Could you check a few things on this model? Use its own coordinates, in mm. A direction names the side the tool comes from. Give positions to 0.01 mm unless a question says otherwise; leave off trailing zeros. Loops run counter-clockwise (first coordinate to the right, second up) from the corner with the lowest first, then second, coordinate; pieces in that order, holes last. Notation, with made-up numbers: (13, 15) - (58, 15) arc R16 ccw to (58, 39) - close; hole circle Ø9 at (6.25, 37). An arc over 180 degrees is marked (long way). Use CSV: the item, a comma, the result in double quotes.
from build123d import *

# Parameters (mm, degrees)
SKETCH_1_W          = 45
SKETCH_1_H          = 39
EXTRUDE_1_DEPTH     = 15
CUT_EXTRUDE_1_DEPTH = 11
SKETCH_3_R          = 1.85
CUT_EXTRUDE_2_DEPTH = 3
SKETCH_4_R          = 1.25
CUT_EXTRUDE_3_DEPTH = 40.575876491
SKETCH_5_R          = 8
CUT_EXTRUDE_4_DEPTH = 12
SKETCH_6_R          = 2.5
EXTRUDE_2_DEPTH     = 1
SKETCH_7_R          = 1.5
EXTRUDE_3_DEPTH     = 1.8
SKETCH_8_W          = 45
SKETCH_8_H          = 15
EXTRUDE_4_DEPTH     = 6
SKETCH_10_R         = 1.5
CUT_EXTRUDE_5_DEPTH = 38.16853512
CUT_EXTRUDE_6_DEPTH = 8.3
SKETCH_12_R         = 4.25
CUT_EXTRUDE_7_DEPTH = 38.16853508
CHAMFER_4_SIZE      = 2
CHAMFER_2_SIZE      = 0.5
CHAMFER_3_SIZE      = 1


with BuildPart() as part:
    # 草图1 → 凸台-拉伸1 (new body)
    with BuildSketch(Plane(origin=(0, 0, 0), x_dir=(1, 0, 0), z_dir=(0, 1, 0))):
        Rectangle(SKETCH_1_W, SKETCH_1_H)
    extrude(amount=EXTRUDE_1_DEPTH)

    # 草图2 → 切除-拉伸1 (cut)
    with BuildSketch(Plane.ZY.offset(22.5)):
        Polygon((-8, 13), (-8, 15), (-6, 15), (-6, 13), (-2.5, 13), (-2.5, 5.65), (-11.5, 5.65), (-11.5, 13), align=None)
        Polygon((6, 2), (6, 0), (8, 0), (8, 2), (11.5, 2), (11.5, 9.35), (2.5, 9.35), (2.5, 2), align=None)
    cut_extrude_1 = extrude(amount=-CUT_EXTRUDE_1_DEPTH, mode=Mode.SUBTRACT)

    # 草图3 → 切除-拉伸2 (cut)
    with BuildSketch(Plane.ZY.offset(11.5)):
        with Locations((-7, 9.325)):
            Circle(SKETCH_3_R)
        with Locations((7, 5.675)):
            Circle(SKETCH_3_R)
    cut_extrude_2 = extrude(amount=-CUT_EXTRUDE_2_DEPTH, mode=Mode.SUBTRACT)

    # 草图4 → 切除-拉伸3 (cut, through all)
    with BuildSketch(Plane.ZY.offset(8.5)):
        with Locations((-7, 9.325)):
            Circle(SKETCH_4_R)
        with Locations((7, 5.675)):
            Circle(SKETCH_4_R)
    extrude(amount=-CUT_EXTRUDE_3_DEPTH, mode=Mode.SUBTRACT)

    # 镜向1: 切除-拉伸1, 切除-拉伸2 across plane
    add(cut_extrude_1.mirror(Plane(origin=(0, 0, 0), x_dir=(0, 0, 1), z_dir=(1, 0, 0))), mode=Mode.SUBTRACT)
    add(cut_extrude_2.mirror(Plane(origin=(0, 0, 0), x_dir=(0, 0, 1), z_dir=(1, 0, 0))), mode=Mode.SUBTRACT)

    # 草图5 → 切除-拉伸4 (cut)
    with BuildSketch(Plane.XZ):
        with Locations(Location((0, 0, 0), (0, 0, 270))):
            Circle(SKETCH_5_R)
    extrude(amount=-CUT_EXTRUDE_4_DEPTH, mode=Mode.SUBTRACT)

    # 草图6 → 凸台-拉伸2 (add)
    with BuildSketch(Plane.XZ.offset(-12)):
        with Locations(Location((0, 0, 0), (0, 0, 270))):
            Circle(SKETCH_6_R)
    extrude(amount=EXTRUDE_2_DEPTH)

    # 草图7 → 凸台-拉伸3 (add)
    with BuildSketch(Plane.XZ.offset(-11)):
        with Locations(Location((0, 0, 0), (0, 0, 270))):
            Circle(SKETCH_7_R)
    extrude(amount=EXTRUDE_3_DEPTH)

    # 草图8 → 凸台-拉伸4 (add)
    with BuildSketch(Plane.XY.offset(19.5)):
        with Locations((0, 7.5)):
            Rectangle(SKETCH_8_W, SKETCH_8_H)
    extrude(amount=EXTRUDE_4_DEPTH)

    # 草图10 → 切除-拉伸5 (cut, through all)
    with BuildSketch(Plane(origin=(0, 15, 0), x_dir=(1, 0, 0), z_dir=(0, 1, 0))):
        with Locations(Location((-19.5, 16.5, 0), (0, 0, 270))):
            Circle(SKETCH_10_R)
        with Locations(Location((19.5, 16.5, 0), (0, 0, 90))):
            Circle(SKETCH_10_R)
        with Locations(Location((19.5, -22.5, 0), (0, 0, 270))):
            Circle(SKETCH_10_R)
        with Locations(Location((-19.5, -22.5, 0), (0, 0, 90))):
            Circle(SKETCH_10_R)
    extrude(amount=-CUT_EXTRUDE_5_DEPTH, mode=Mode.SUBTRACT)

    # 草图11 → 切除-拉伸6 (cut)
    with BuildSketch(Plane(origin=(0, 15, 0), x_dir=(1, 0, 0), z_dir=(0, 1, 0))):
        with BuildLine():
            Line((-16.5, 16.5), (-16.5, 19.5))
            Line((-16.5, 19.5), (-22.5, 19.5))
            Line((-22.5, 19.5), (-22.5, 13.5))
            Line((-22.5, 13.5), (-19.5, 13.5))
            ThreePointArc((-19.5, 13.5), (-17.378679656, 14.378679656), (-16.5, 16.5))
        make_face()
        with BuildLine():
            Line((22.5, 19.5), (22.5, 13.5))
            Line((22.5, 13.5), (19.5, 13.5))
            ThreePointArc((19.5, 13.5), (17.378679656, 14.378679656), (16.5, 16.5))
            Line((16.5, 16.5), (16.5, 19.5))
            Line((16.5, 19.5), (22.5, 19.5))
        make_face()
        with BuildLine():
            Line((16.5, -25.5), (22.5, -25.5))
            Line((22.5, -25.5), (22.5, -19.5))
            Line((22.5, -19.5), (19.5, -19.5))
            ThreePointArc((19.5, -19.5), (17.378679656, -20.378679656), (16.5, -22.5))
            Line((16.5, -22.5), (16.5, -25.5))
        make_face()
        with BuildLine():
            Line((-22.5, -25.5), (-22.5, -19.5))
            Line((-22.5, -19.5), (-19.5, -19.5))
            ThreePointArc((-19.5, -19.5), (-17.378679656, -20.378679656), (-16.5, -22.5))
            Line((-16.5, -22.5), (-16.5, -25.5))
            Line((-16.5, -25.5), (-22.5, -25.5))
        make_face()
    extrude(amount=-CUT_EXTRUDE_6_DEPTH, mode=Mode.SUBTRACT)

    # 草图12 → 切除-拉伸7 (cut, through all)
    with BuildSketch(Plane.XZ):
        with Locations(Location((0, 17.5, 0), (0, 0, 270))):
            Circle(SKETCH_12_R)
    extrude(amount=-CUT_EXTRUDE_7_DEPTH, mode=Mode.SUBTRACT)

    # 倒角4
    chamfer_4_edges = [part.edges().sort_by_distance(p)[0] for p in [
        (0, 0, 21.75),
    ]]
    chamfer(chamfer_4_edges, length=CHAMFER_4_SIZE)

    # 倒角2
    chamfer_2_edges = [part.edges().sort_by_distance(p)[0] for p in [
        (0, 9.2, 1.5),
    ]]
    chamfer(chamfer_2_edges, length=CHAMFER_2_SIZE)

    # 倒角3
    chamfer_3_edges = [part.edges().sort_by_distance(p)[0] for p in [
        (22.5, 3.35, 25.5),
        (-22.5, 3.35, 25.5),
        (-22.5, 3.35, -19.5),
        (22.5, 3.35, -19.5),
    ]]
    chamfer(chamfer_3_edges, length=CHAMFER_3_SIZE)


solid = part.part
1) Suppose I cut it at D-D (z = -9.5). Please give me the cut outline in (x, y), plus the area to 3 significant figures.
Answer below:
outline,"(-22.5, 0) - (22.5, 0) - (22.5, 5.65) - (11.5, 5.65) - (11.5, 13) - (22.5, 13) - (22.5, 15) - (-22.5, 15) - (-22.5, 13) - (-11.5, 13) - (-11.5, 5.65) - (-22.5, 5.65) - close"
area,"513 mm2"
2) We'd pull the mould along Z, two halves only. Please class faces 1 (the flat face through (0, 8, 25.5)), 2 (the cylindrical face through (4.214, 8.409, 18.053)), 3 (the cylindrical face through (-17.4, 10.91, -14.36)), 4 (the flat face through (22.5, 11, 3)): +Z half, -Z half, draft (parallel to the pull), parting line (faces both ways), or undercut.
Answer below:
face 1,"+Z half"
face 2,"undercut"
face 3,"-Z half"
face 4,"draft"
3) I'm going to push flat-ended pins straight in: P1, Ø1.5, axis at x = 21, y = 12.5, coming from the -Z side; P2, Ø4.5, axis at y = 5.675, z = 7, coming from the -X side; P3, Ø2, axis at y = 9.325, z = -7, coming from the +X side; P4, Ø1, axis at x = 2, z = -3.5, coming from the -Y side. Where does each tip first touch, or does it pass through?
Answer below:
P1,"stops at z = -13.5"
P2,"stops at x = -11.5"
P3,"passes through"
P4,"stops at y = 12"
4) Suppose I cut it at B-B (y = 3). Please give me the cut outline in (x, z).
Answer below:
outline,"(-22.5, -18.5) - (-21.5, -19.5) - (21.5, -19.5) - (22.5, -18.5) - (22.5, 2.5) - (11.5, 2.5) - (11.5, 11.5) - (22.5, 11.5) - (22.5, 24.5) - (21.5, 25.5) - (-21.5, 25.5) - (-22.5, 24.5) - (-22.5, 11.5) - (-11.5, 11.5) - (-11.5, 2.5) - (-22.5, 2.5) - close; hole circle Ø3 at (-19.5, -16.5); hole circle Ø3 at (-19.5, 22.5); hole circle Ø16 at (0, 0); hole circle Ø8.5 at (0, 17.5); hole circle Ø3 at (19.5, -16.5); hole circle Ø3 at (19.5, 22.5)"
5) I need wall thicknesses on line 1 along Z through (x, y) = (14, 7.25); line 2 along X through (y, z) = (1.5, -16.5); line 3 along Z through (x, y) = (-1, 2.25). Which ranges of each line are inside material? Lowest first, please.
Answer below:
line 1,"z = -19.5 to -11.5, -2.5 to 2.5, 11.5 to 25.5"
line 2,"x = -22.5 to -21, -18 to 18, 21 to 22.5"
line 3,"z = -19.5 to -7.94, 7.94 to 13.37, 21.63 to 25.5"
6) Suppose I cut it at C-C (z = 7). Please give me the cut outline in (x, y) (3 decimals).
Answer below:
outline,"(-22.5, 9.35) - (-11.5, 9.35) - (-11.5, 7.525) - (-8.5, 7.525) - (-8.5, 6.925) - (-3.873, 6.925) - (-3.873, 12) - (3.873, 12) - (3.873, 6.925) - (8.5, 6.925) - (8.5, 7.525) - (11.5, 7.525) - (11.5, 9.35) - (22.5, 9.35) - (22.5, 15) - (-22.5, 15) - close; (-11.5, 0) - (-3.873, 0) - (-3.873, 4.425) - (-8.5, 4.425) - (-8.5, 3.825) - (-11.5, 3.825) - close; (3.873, 0) - (11.5, 0) - (11.5, 3.825) - (8.5, 3.825) - (8.5, 4.425) - (3.873, 4.425) - close"
7) Suppose I cut it at A-A (z = 17.5). Please give me the cut outline in (x, y), plus the area to 4 significant figures.
Answer below:
outline,"(-22.5, 0) - (-6.25, 0) - (-4.25, 2) - (-4.25, 15) - (-22.5, 15) - close; (4.25, 2) - (6.25, 0) - (22.5, 0) - (22.5, 15) - (4.25, 15) - close"
area,"543.5 mm2"
8) Which directions (+Z, -Z, +X, -X, +Y, -Y) give clear straight access to the entire face, cutting with the end or side of a thin tool? Please do faces 5 (the flat face through (-16.5, 11, -18)), 6 (the flat face through (-8.5, 11, -7)), 7 (the flat face through (21, 6.7, -18)), 8 (the flat face through (-17, 14, -6)), 9 (the flat face through (0, 9.2, 0)).
Answer below:
face 5,"-Z, -X, +Y"
face 6,"-X"
face 7,"-Z, +X, +Y"
face 8,"-X, +Y"
face 9,"-Y"
